Source: CAD feature listing. Evaluate the final solid. Frame: model axes, mm. A direction names the side the tool comes from. Give positions to 0.01 mm unless a question says otherwise; leave off trailing zeros. Loops run counter-clockwise (first coordinate to the right, second up) from the corner with the lowest first, then second, coordinate; pieces in that order, holes last. Notation, with made-up numbers: M -0.75,-26.75 L 9.25,-26.75 A14 cw 9.25,0.25 Z; hole C 18.5,12.5 d11. An arc over 180 degrees is marked long. Put each result on its own line as item: value.
Autodesk Inventor part; units mm, degrees
ref_plane "YZ Plane" through (0, 0, 0) normal (1, 0, 0) x (0, 1, 0)
ref_plane "XZ Plane" through (0, 0, 0) normal (0, 1, 0) x (-1, 0, 0)
ref_plane "XY Plane" through (0, 0, 0) normal (0, 0, 1) x (1, 0, 0)
sketch "Sketch1" plane through (0, 0, 0) normal (1, 0, 0) x (0, 1, 0)
  line L0 (0, 0) -> (30, 0)
  line L1 (30, 0) -> (30, 32)
  line L2 (30, 32) -> (0, 32)
  line L3 (0, 32) -> (0, 0)
  dimension "d0" = 30
  dimension "d1" = 32
extrude "Extrusion1" add sketch "Sketch1" along normal blind 85
sketch "Sketch2" plane through (0, 30, 32) normal (0, 1, 0) x (1, 0, 0)
  line L0 (0, 32) -> (0, 0)
  line L1 (0, 0) -> (85, 0)
  line L2 (85, 32) -> (85, 0)
  line L3 (0, 32) -> (85, 32)
  line L4 (5, 5) -> (80, 5)
  line L5 (80, 5) -> (80, 27)
  line L6 (80, 27) -> (5, 27)
  line L7 (5, 27) -> (5, 5)
  line L8 (5, 5) -> (80, 27) construction
  line L9 (80, 5) -> (5, 27) construction
  point P0 (42.5, 16)
  dimension "d12" = 75
  dimension "d13" = 22
extrude "Extrusion2" cut sketch "Sketch2" against normal blind 28 contours L7 L6 L5 L4
sketch "Sketch3" plane through (0, 0, 0) normal (-1, 0, 0) x (0, 0, 1)
  circle A0 centre (21.6569, 19.6569) radius 1.85
  circle A1 centre (21.6569, 8.3431) radius 1.85
  circle A2 centre (10.3431, 8.3431) radius 1.85
  circle A3 centre (10.3431, 19.6569) radius 1.85
  point P0 (0, 0)
extrude "Extrusion3" cut sketch "Sketch3" against normal through all
sketch "Sketch4" plane through (0, 0, 0) normal (0, -1, 0) x (1, 0, 0)
  circle A0 centre (22, 16) radius 1.85
  circle A1 centre (70, 16) radius 1.85
  point P0 (0, 0)
extrude "Extrusion5" cut sketch "Sketch4" against normal through all
properties part number "sidebracket"
1. Section query D-D (z = 7). Output: boundary loops of the cut face in (x, y).
Found:
outline: M 0,0 L 85,0 L 85,30 L 80,30 L 80,2 L 5,2 L 5,30 L 0,30 Z
2. Section query C-C (z = 16). Output: boundary loops of the cut face in (x, y), plus the area to 3 significant figures.
Found:
outline: M 0,0 L 20.15,0 L 20.15,2 L 5,2 L 5,30 L 0,30 Z; M 23.85,0 L 68.15,0 L 68.15,2 L 23.85,2 Z; M 71.85,0 L 85,0 L 85,30 L 80,30 L 80,2 L 71.85,2 Z
area: 435 mm^2
3. Contact query for flat-ended pins moving along their axis: P1, Ø8, axis at x = 76, z = 3.5, coming from the -Y side; P2, Ø3, axis at y = 8.34, z = 21.66, coming from the -X side; P3, Ø6, axis at x = 22, z = 16, coming from the +Y side. Output: stop coordinate, or through.
Found:
P1: y = 0
P2: through
P3: y = 2
4. Section query A-A (x = 22). Output: boundary loops of the cut face in (y, z), plus the area to 3 significant figures.
Found:
outline: M 0,0 L 30,0 L 30,5 L 2,5 L 2,14.15 L 0,14.15 Z; M 0,17.85 L 2,17.85 L 2,27 L 30,27 L 30,32 L 0,32 Z
area: 337 mm^2
5. Draft query along Z for faces 3 (the flat face through (5, 16, 16)), 4 (the flat face through (42, 15, 0)), 5 (the cylindrical face through (2.46, 9.9, 11.34)), 6 (the flat face through (42, 15, 32)). Return one class per face: pulls with the +Z half, pulls with the -Z half, needs draft (parallel to the pull), parting line crosses it, or undercut.
Found:
face 3: undercut
face 4: pulls with the -Z half
face 5: undercut
face 6: pulls with the +Z half
6. Section query B-B (y = 26.5). Output: boundary loops of the cut face in (x, z), plus the area to 3 significant figures.
Found:
outline: M 0,0 L 85,0 L 85,32 L 0,32 Z; hole M 5,5 L 80,5 L 80,27 L 5,27 Z
area: 1,070 mm^2
7. Material intervals for line 1 (X direction, y = 14.25, z = 26.5); line 2 (Z direction, x = 13.5, y = 18.75); line 3 (Z direction, x = 22, y = 1.5), sorted ascending. Write a range as from..to.
Found:
line 1: 0..5, 80..85
line 2: 0..5, 27..32
line 3: 0..14.15, 17.85..32
8. Access query for faces 1 (the flat face through (80, 16, 16)), 2 (the cylindrical face through (2.46, 8.9, 23.42)). Directions: +Z, -Z, +X, -X, +Y, -Y. A direction counts if a zero-diameter tool reaches every point of the face in a straight line with its end or side. Return the directions, or none.
Found:
face 1: +Y
face 2: +X, -X
